Autodesk Fusion 360 part; units mm, degrees
sketch "Sketch1" plane through (0, 0, 0) normal (0, 1, 0) x (1, 0, 0)
  line L0 (2, 0) -> (98.5, 0) construction
  line L1 (100.5, 2) -> (100.5, 98.5) construction
  line L2 (98.5, 100.5) -> (2, 100.5) construction
  line L3 (0, 98.5) -> (0, 2) construction
  circle A0 centre (5, 95.5) radius 1.6 construction
  circle A1 centre (95.5, 95.5) radius 1.6 construction
  circle A2 centre (5, 5) radius 1.6 construction
  circle A3 centre (95.5, 5) radius 1.6 construction
  line L4 (99.5, 97.5) -> (99.5, 3)
  line L5 (97.5, 1) -> (3, 1)
  line L6 (1, 3) -> (1, 97.5)
  line L7 (102, 98.5) -> (102, 0.5)
  line L8 (100, -1.5) -> (0.5, -1.5)
  line L9 (-1.5, 0.5) -> (-1.5, 98.5)
  arc A4 (100, -1.5) -> (102, 0.5) centre (100, 0.5) ccw
  arc A5 (-1.5, 0.5) -> (0.5, -1.5) centre (0.5, 0.5) ccw
  arc A6 (0.5, 100.5) -> (-1.5, 98.5) centre (0.5, 98.5) ccw
  arc A7 (102, 98.5) -> (100, 100.5) centre (100, 98.5) ccw
  arc A8 (97.5, 1) -> (99.5, 3) centre (97.5, 3) ccw
  arc A9 (99.5, 97.5) -> (97.5, 99.5) centre (97.5, 97.5) ccw
  arc A10 (3, 99.5) -> (1, 97.5) centre (3, 97.5) ccw
  arc A11 (1, 3) -> (3, 1) centre (3, 3) ccw
  line L10 (99.5, 88.5) -> (91.5, 88.5)
  line L11 (88.5, 91.5) -> (88.5, 99.5)
  line L12 (99.5, 12) -> (91.5, 12)
  line L13 (88.5, 9) -> (88.5, 1)
  line L14 (1, 12) -> (9, 12)
  line L15 (12, 9) -> (12, 1)
  line L16 (12, 99.5) -> (12, 91.5)
  line L17 (9, 88.5) -> (1, 88.5)
  arc A12 (88.5, 91.5) -> (91.5, 88.5) centre (91.5, 91.5) ccw
  arc A13 (9, 88.5) -> (12, 91.5) centre (9, 91.5) ccw
  arc A14 (12, 9) -> (9, 12) centre (9, 9) ccw
  arc A15 (91.5, 12) -> (88.5, 9) centre (91.5, 9) ccw
  circle A16 centre (95.5, 95.5) radius 3
  circle A17 centre (95.5, 5) radius 3
  circle A18 centre (5, 5) radius 3
  circle A19 centre (5, 95.5) radius 3
  line L18 (3, 99.5) -> (12, 99.5)
  line L19 (88.5, 99.5) -> (97.5, 99.5)
  line L20 (88.5, 99.5) -> (88.5, 100.5)
  line L21 (12, 99.5) -> (12, 100.5)
  line L22 (0.5, 100.5) -> (12, 100.5)
  line L23 (88.5, 100.5) -> (100, 100.5)
  arc A20 (98.5, 0) -> (100.5, 2) centre (98.5, 2) ccw construction
  arc A21 (100.5, 98.5) -> (98.5, 100.5) centre (98.5, 98.5) ccw construction
  arc A22 (2, 100.5) -> (0, 98.5) centre (2, 98.5) ccw construction
  arc A23 (0, 2) -> (2, 0) centre (2, 2) ccw construction
  point P0 (100.5, 0)
  point P1 (0, 100.5)
  dimension "d1" = 100.5
  dimension "d2" = 100.5
  dimension "d3" = 3.2
  dimension "d4" = 5
  dimension "d5" = 5
  dimension "d6" = 3.2
  dimension "d7" = 3.2
  dimension "d8" = 3.2
  dimension "d9" = 5
  dimension "d10" = 1
  dimension "d11" = 1
  dimension "d12" = 1
  dimension "d13" = 1
  dimension "d14" = 2.5
  dimension "d15" = 2.5
  dimension "d16" = 2.5
  dimension "d17" = 2
  dimension "d18" = 2
  dimension "d19" = 2
  dimension "d20" = 2
  dimension "d21" = 2
  dimension "d22" = 2
  dimension "d23" = 2
  dimension "d24" = 2
  dimension "d27" = 12
  dimension "d28" = 12
  dimension "d29" = 12
  dimension "d30" = 12
  dimension "d31" = 12
  dimension "d32" = 12
  dimension "d33" = 12
  dimension "d34" = 12
  dimension "d35" = 3
  dimension "d36" = 3
  dimension "d37" = 6
  dimension "d38" = 6
  dimension "d39" = 6
  dimension "d40" = 6
  dimension "d43" = 2
  dimension "d44" = 2
  dimension "d45" = 2
  dimension "d46" = 2
extrude "Extrude1" add sketch "Sketch1" along normal blind 4
sketch "Sketch2" plane through (0, 4, 0) normal (0, 1, 0) x (-1, 0, 0)
  circle A0 centre (-95.5, -5) radius 3
  circle A1 centre (-5, -5) radius 3
  circle A2 centre (-95.5, -95.5) radius 3
  circle A3 centre (-5, -95.5) radius 3
  arc A4 (-88.5, -91.5) -> (-91.5, -88.5) centre (-91.5, -91.5) ccw
  line L0 (-91.5, -88.5) -> (-99.5, -88.5)
  line L1 (-99.5, -88.5) -> (-99.5, -12)
  line L2 (-99.5, -12) -> (-91.5, -12)
  arc A5 (-91.5, -12) -> (-88.5, -9) centre (-91.5, -9) ccw
  line L3 (-88.5, -9) -> (-88.5, -1)
  line L4 (-88.5, -1) -> (-12, -1)
  line L5 (-12, -1) -> (-12, -9)
  arc A6 (-12, -9) -> (-9, -12) centre (-9, -9) ccw
  line L6 (-9, -12) -> (-1, -12)
  line L7 (-1, -12) -> (-1, -88.5)
  line L8 (-1, -88.5) -> (-9, -88.5)
  arc A7 (-9, -88.5) -> (-12, -91.5) centre (-9, -91.5) ccw
  line L9 (-12, -91.5) -> (-12, -100.5)
  line L10 (-12, -100.5) -> (-0.5, -100.5)
  arc A8 (-0.5, -100.5) -> (1.5, -98.5) centre (-0.5, -98.5) ccw
  line L11 (1.5, -98.5) -> (1.5, -0.5)
  arc A9 (1.5, -0.5) -> (-0.5, 1.5) centre (-0.5, -0.5) ccw
  line L12 (-0.5, 1.5) -> (-100, 1.5)
  arc A10 (-100, 1.5) -> (-102, -0.5) centre (-100, -0.5) ccw
  line L13 (-102, -0.5) -> (-102, -98.5)
  arc A11 (-102, -98.5) -> (-100, -100.5) centre (-100, -98.5) ccw
  line L14 (-100, -100.5) -> (-88.5, -100.5)
  line L15 (-88.5, -100.5) -> (-88.5, -91.5)
  arc A12 (0, -2) -> (-2, 0) centre (-2, -2) ccw
  line L16 (-2, 0) -> (-98.5, 0)
  arc A13 (1.5, -0.5) -> (-0.5, 1.5) centre (-0.5, -0.5) ccw
  line L17 (-0.5, 1.5) -> (-100, 1.5)
  arc A14 (-98.5, 0) -> (-100.5, -2) centre (-98.5, -2) ccw
  line L18 (-100.5, -2) -> (-100.5, -98.5)
  arc A15 (-100, 1.5) -> (-102, -0.5) centre (-100, -0.5) ccw
  line L19 (-102, -98.5) -> (-102, -0.5)
  line L20 (-98.5, -100.5) -> (-2, -100.5)
  line L21 (-100, -100.5) -> (-88.5, -100.5)
  arc A16 (-102, -98.5) -> (-100, -100.5) centre (-100, -98.5) ccw
  line L22 (-102, -0.5) -> (-102, -98.5)
  line L23 (0, -98.5) -> (0, -2)
  arc A17 (-0.5, -100.5) -> (1.5, -98.5) centre (-0.5, -98.5) ccw
  line L24 (1.5, -98.5) -> (1.5, -0.5)
  line L25 (0, -98.5) -> (0, -100.5)
  line L26 (-100.5, -98.5) -> (-100.5, -100.5)
extrude "Extrude3" add sketch "Sketch2" along normal blind 1.5 contours A8 L11 A9 L12 A10 L13 A11 A12 L16 A13 L17 A14 L18 A15 L19 A16 L22 L23 A17 L24 L25 L26
fillet "Fillet2" radius 0.3 7 edges at (-1.0811, 5.5, -99.7247) (-1.5, 5.5, -49.5) (-0.9142, 5.5, 0.9142) (50.25, 5.5, 1.5) (101.4142, 5.5, 0.9142) (102, 5.5, -49.5) (101.5811, 5.5, -99.7247)
extrude "Extrude2" add sketch "Sketch2" along normal blind 1.5 contours A8 L11 A9 L12 A10 L13 A11 A12 L16 A13 L17 A14 L18 A15 L19 A16 L22 L23 A17 L24 L25 L26
fillet "Fillet1" radius 0.3 7 edges at (-1.0811, 5.5, -99.7247) (-1.5, 5.5, -49.5) (-0.9142, 5.5, 0.9142) (50.25, 5.5, 1.5) (101.4142, 5.5, 0.9142) (102, 5.5, -49.5) (101.5811, 5.5, -99.7247)
fillet "Fillet3" radius 2 1 edges at (12, 2, -100.5)
fillet "Fillet3" radius 2 1 edges at (88.5, 2, -100.5)
fillet "Fillet3" radius 2 1 edges at (99.5, 2, -88.5)
fillet "Fillet3" radius 2 1 edges at (99.5, 2, -12)
fillet "Fillet3" radius 2 1 edges at (88.5, 2, -1)
fillet "Fillet3" radius 2 1 edges at (12, 2, -1)
fillet "Fillet3" radius 2 1 edges at (1, 2, -12)
fillet "Fillet3" radius 2 1 edges at (1, 2, -88.5)
The model under review builds one solid part; all positions refer to its coordinate system, in mm. A direction names the side the tool comes from. Round coordinates to 2 decimals unless told otherwise and drop trailing zeros. Write each loop counter-clockwise with the first axis right and the second up, starting at its lowest first coordinate (ties: lowest second). Pieces come first, ordered by that corner, then holes.
(1) We need section B-B on z = -80. Give the boundary of the cut face in (x, y), and give its area (3 significant figures).
(2) We need section D-D on x = 54. Give the boundary of the cut face in (y, z), and give its area (3 significant figures).
(3) Wall thickness on L1, parallel to X at y = 2.1, z = -95.5; L2, parallel to Z at x = 95.5, y = 1.55; L3, parallel to Z at x = 93, y = 1.4: over which ranges is each line inside the solid? List them lowest first.
(4) We need section A-A on x = 95.5. Give the boundary of the cut face in (y, z).
(5) We need section C-C on z = -5. Give the boundary of the cut face in (x, y), and give its area (3 significant figures).
(6) Mouldability with a two-part tool opening along Z and no side actions: class faces 1 (the flat face through (6, 2, -88.5)), 2 (the flat face through (5, 2, -100.5)), 3 (the flat face through (12, 2, -6)) as +Z half, -Z half, draft (parallel to the pull), parting line (faces both ways), or undercut.
(7) Machinability: for faces 4 (the flat face through (88.5, 2, -95)), 5 (the flat face through (95, 2, -12)), 6 (the flat face through (50, 0, -0.6)), which of the approach directions +Z, -Z, +X, -X, +Y, -Y give a long, thin tool a straight path to every point of the face, cutting with its end or side? Answer none if there is none.
Findings below:
1. outline: (-1.5, 0) - (1, 0) - (1, 4) - (0, 4) - (0, 5.5) - (-1.2, 5.5) arc R0.3 ccw to (-1.5, 5.2) - close; (99.5, 0) - (102, 0) - (102, 5.2) arc R0.3 ccw to (101.7, 5.5) - (100.5, 5.5) - (100.5, 4) - (99.5, 4) - close
1. area: 24.5 mm2
2. outline: (0, -1) - (4, -1) - (4, 0) - (5.5, 0) - (5.5, 1.2) arc R0.3 ccw to (5.2, 1.5) - (0, 1.5) - close
2. area: 12.2 mm2
3. L1: x = -1.5 to 2, 8 to 12, 88.5 to 92.5, 98.5 to 102
3. L2: z = -100.5 to -98.5, -92.5 to -88.5, -12 to -8, -2 to 1.5
3. L3: z = -100.5 to -97.16, -93.84 to -88.5, -12 to -6.66, -3.34 to 1.5
4. outline: (0, -100.5) - (4, -100.5) - (4, -98.5) - (0, -98.5) - close; (0, -92.5) - (4, -92.5) - (4, -88.5) - (0, -88.5) - close; (0, -12) - (4, -12) - (4, -8) - (0, -8) - close; (0, -2) - (4, -2) - (4, 0) - (5.5, 0) - (5.5, 1.2) arc R0.3 ccw to (5.2, 1.5) - (0, 1.5) - close
5. outline: (-1.5, 0) - (2, 0) - (2, 4) - (0, 4) - (0, 5.5) - (-1.2, 5.5) arc R0.3 ccw to (-1.5, 5.2) - close; (8, 0) - (12, 0) - (12, 4) - (8, 4) - close; (88.5, 0) - (92.5, 0) - (92.5, 4) - (88.5, 4) - close; (98.5, 0) - (102, 0) - (102, 5.2) arc R0.3 ccw to (101.7, 5.5) - (100.5, 5.5) - (100.5, 4) - (98.5, 4) - close
5. area: 64.5 mm2
6. face 1: undercut
6. face 2: -Z half
6. face 3: draft
7. face 4: -Z, +Y, -Y
7. face 5: +Y, -Y
7. face 6: +Z, -Z, +X, -X, -Y
